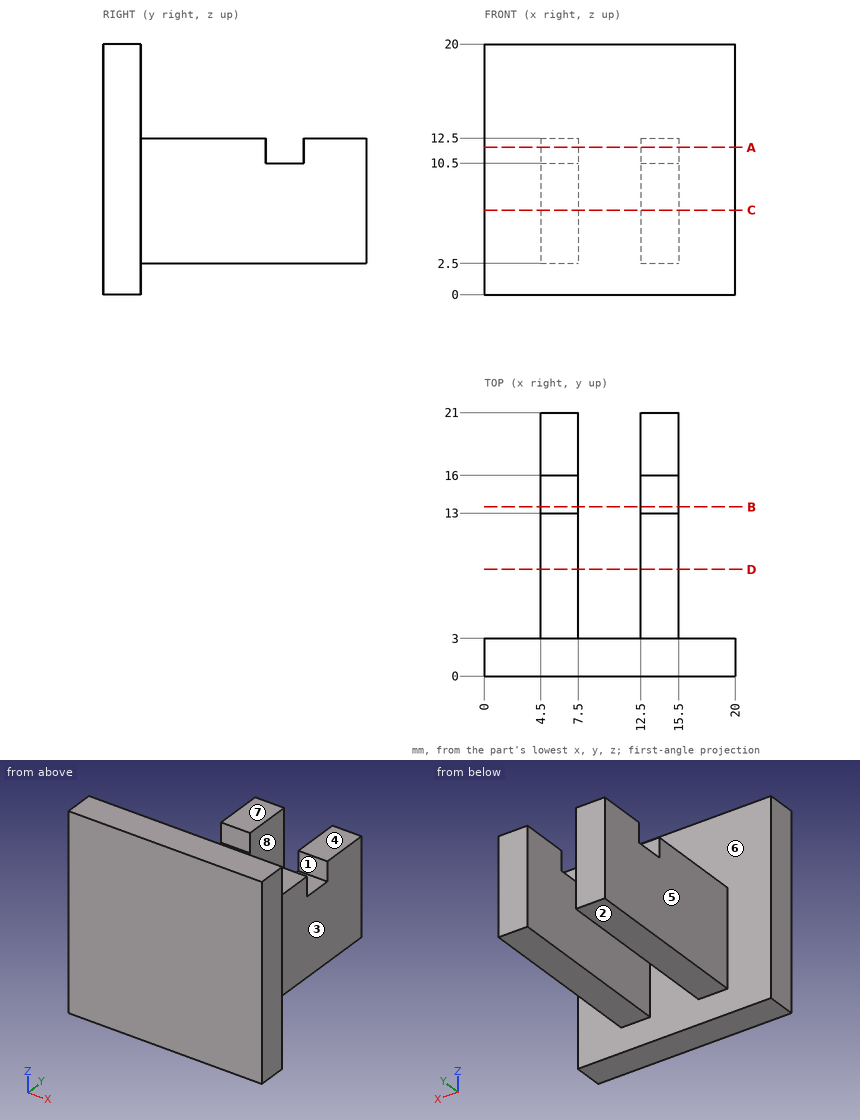
The figure shows three views and two pictorial views of one solid part (mm, origin at its lowest corner). Answer the questions. A direction names the side the tool comes from. Round coordinates to 2 decimals unless told otherwise and drop trailing zeros. Loops run counter-clockwise (first coordinate to the right, second up) from the corner with the lowest first, then second, coordinate; pieces in that order, holes last. Notation, with made-up numbers: (-4.5, -5) - (52.5, -5) arc R19 ccw to (52.5, 14) - close; hole circle Ø6 at (-22.5, -19.75). An arc over 180 degrees is marked (long way). Use one line per item in the form item = value. Start each with the question number.
(1) Flat-ended cylindrical pins translate along their axes: P1, Ø5, axis at x = 4, y = 16.5, coming from the -Z side; P2, Ø3.5, axis at x = 14, y = 6, coming from the +Z side; P3, Ø3, axis at y = 9.5, z = 9, coming from the -X side. Find the tip coordinate at first contact, or state that the pin passes through.
(2) Find section B-B on y = 13.5. Determine the outline of the cut face in (x, z).
(3) Find section A-A on z = 11.75. Determine the outline of the cut face in (x, y), and give its area (3 significant figures).
(4) Which of the six approach directions +Z, -Z, +X, -X, +Y, -Y give full straight-line access (tool end or side, diameter ignored) to the marked faces 1, 2, 3 and 4?
(5) Find section D-D on y = 8.5. Determine the outline of the cut face in (x, z).
(6) Consider line 1 (X direction, y = 7.25, z = 9.5); line 2 (Y direction, x = 1.25, z = 4.25); line 3 (Z direction, x = 7, y = 19.25). Determine where each line is inside the solid, lowest interval first.
(7) Find section C-C on z = 6.75. Determine the outline of the cut face in (x, y), and give its area (3 significant figures).
(8) Determine the mould class of the marked faces 5, 6, 7 and 8 for opening direction X: +X half, -X half, draft (parallel to the pull), parting line (faces both ways), or undercut.
Answer list:
q1.P1 = 2.5
q1.P2 = 12.5
q1.P3 = 4.5
q2.outline = (4.5, 2.5) - (7.5, 2.5) - (7.5, 10.5) - (4.5, 10.5) - close; (12.5, 2.5) - (15.5, 2.5) - (15.5, 10.5) - (12.5, 10.5) - close
q3.outline = (0, 0) - (20, 0) - (20, 3) - (15.5, 3) - (15.5, 13) - (12.5, 13) - (12.5, 3) - (7.5, 3) - (7.5, 13) - (4.5, 13) - (4.5, 3) - (0, 3) - close; (4.5, 16) - (7.5, 16) - (7.5, 21) - (4.5, 21) - close; (12.5, 16) - (15.5, 16) - (15.5, 21) - (12.5, 21) - close
q3.area = 150 mm^2
q4.face_1 = +Z, +X, -X
q4.face_2 = -Z, +X, -X, +Y
q4.face_3 = +Z, -Z, +X, +Y
q4.face_4 = +Z, +X, -X, +Y
q5.outline = (4.5, 2.5) - (7.5, 2.5) - (7.5, 12.5) - (4.5, 12.5) - close; (12.5, 2.5) - (15.5, 2.5) - (15.5, 12.5) - (12.5, 12.5) - close
q6.line_1 = 4.5 to 7.5, 12.5 to 15.5
q6.line_2 = 0 to 3
q6.line_3 = 2.5 to 12.5
q7.outline = (0, 0) - (20, 0) - (20, 3) - (15.5, 3) - (15.5, 21) - (12.5, 21) - (12.5, 3) - (7.5, 3) - (7.5, 21) - (4.5, 21) - (4.5, 3) - (0, 3) - close
q7.area = 168 mm^2
q8.face_5 = -X half
q8.face_6 = undercut
q8.face_7 = draft
q8.face_8 = undercut
